Autodesk Inventor part; units mm, degrees
ref_plane "YZ Plane" through (0, 0, 0) normal (1, 0, 0) x (0, 1, 0)
ref_plane "XZ Plane" through (0, 0, 0) normal (0, 1, 0) x (-1, 0, 0)
ref_plane "XY Plane" through (0, 0, 0) normal (0, 0, 1) x (1, 0, 0)
sketch "Sketch1" plane through (0, 0, 0) normal (0, 0, 1) x (1, 0, 0)
  circle A0 centre (0, 0) radius 30
  circle A1 centre (0, 0) radius 22
  dimension "d0" = 60
  dimension "d1" = 44
extrude "Extrusion1" add sketch "Sketch1" against normal blind 1.17
sketch "Sketch2" plane through (0, 0, 0) normal (0, 0, 1) x (1, 0, 0)
  circle A0 centre (0, 0) radius 26 construction
  line L0 (-1.8, 24.6) -> (1.8, 24.6)
  line L1 (1.8, 24.6) -> (1.8, 27.4)
  line L2 (1.8, 27.4) -> (-1.8, 27.4)
  line L3 (-1.8, 27.4) -> (-1.8, 24.6)
  line L4 (-1.8, 24.6) -> (1.8, 27.4) construction
  line L5 (1.8, 24.6) -> (-1.8, 27.4) construction
  line L6 (12.789, 24.299) -> (9.5002, 25.7633)
  line L7 (11.6501, 21.7411) -> (12.789, 24.299)
  line L8 (8.3613, 23.2053) -> (11.6501, 21.7411)
  circle A1 centre (0, 0) radius 26 construction
  line L9 (9.5002, 25.7633) -> (8.3613, 23.2053)
  line L10 (21.5666, 16.9965) -> (19.1577, 19.6718)
  line L11 (19.4858, 15.123) -> (21.5666, 16.9965)
  line L12 (17.0769, 17.7983) -> (19.4858, 15.123)
  circle A2 centre (0, 0) radius 26 construction
  line L13 (19.1577, 19.6718) -> (17.0769, 17.7983)
  line L14 (26.6152, 6.7552) -> (25.5027, 10.179)
  line L15 (23.9522, 5.8899) -> (26.6152, 6.7552)
  line L16 (22.8398, 9.3137) -> (23.9522, 5.8899)
  circle A3 centre (0, 0) radius 26 construction
  line L17 (25.5027, 10.179) -> (22.8398, 9.3137)
  line L18 (27.0617, -4.6542) -> (27.4381, -1.0739)
  line L19 (24.2771, -4.3615) -> (27.0617, -4.6542)
  line L20 (24.6534, -0.7813) -> (24.2771, -4.3615)
  circle A4 centre (0, 0) radius 26 construction
  line L21 (27.4381, -1.0739) -> (24.6534, -0.7813)
  line L22 (22.8291, -15.2588) -> (24.6291, -12.1412)
  line L23 (20.4042, -13.8588) -> (22.8291, -15.2588)
  line L24 (22.2042, -10.7412) -> (20.4042, -13.8588)
  circle A5 centre (0, 0) radius 26 construction
  line L25 (24.6291, -12.1412) -> (22.2042, -10.7412)
  line L26 (14.6491, -23.2251) -> (17.5615, -21.1091)
  line L27 (13.0033, -20.9598) -> (14.6491, -23.2251)
  line L28 (15.9157, -18.8438) -> (13.0033, -20.9598)
  circle A6 centre (0, 0) radius 26 construction
  line L29 (17.5615, -21.1091) -> (15.9157, -18.8438)
  line L30 (3.9361, -27.1755) -> (7.4574, -26.427)
  line L31 (3.354, -24.4367) -> (3.9361, -27.1755)
  line L32 (6.8753, -23.6882) -> (3.354, -24.4367)
  circle A7 centre (0, 0) radius 26 construction
  line L33 (7.4574, -26.427) -> (6.8753, -23.6882)
  line L34 (-7.4574, -26.427) -> (-3.9361, -27.1755)
  line L35 (-6.8753, -23.6882) -> (-7.4574, -26.427)
  line L36 (-3.354, -24.4367) -> (-6.8753, -23.6882)
  circle A8 centre (0, 0) radius 26 construction
  line L37 (-3.9361, -27.1755) -> (-3.354, -24.4367)
  line L38 (-17.5615, -21.1091) -> (-14.6491, -23.2251)
  line L39 (-15.9157, -18.8438) -> (-17.5615, -21.1091)
  line L40 (-13.0033, -20.9598) -> (-15.9157, -18.8438)
  circle A9 centre (0, 0) radius 26 construction
  line L41 (-14.6491, -23.2251) -> (-13.0033, -20.9598)
  line L42 (-24.6291, -12.1412) -> (-22.8291, -15.2588)
  line L43 (-22.2042, -10.7412) -> (-24.6291, -12.1412)
  line L44 (-20.4042, -13.8588) -> (-22.2042, -10.7412)
  circle A10 centre (0, 0) radius 26 construction
  line L45 (-22.8291, -15.2588) -> (-20.4042, -13.8588)
  line L46 (-27.4381, -1.0739) -> (-27.0617, -4.6542)
  line L47 (-24.6534, -0.7813) -> (-27.4381, -1.0739)
  line L48 (-24.2771, -4.3615) -> (-24.6534, -0.7813)
  circle A11 centre (0, 0) radius 26 construction
  line L49 (-27.0617, -4.6542) -> (-24.2771, -4.3615)
  line L50 (-25.5027, 10.179) -> (-26.6152, 6.7552)
  line L51 (-22.8398, 9.3137) -> (-25.5027, 10.179)
  line L52 (-23.9522, 5.8899) -> (-22.8398, 9.3137)
  circle A12 centre (0, 0) radius 26 construction
  line L53 (-26.6152, 6.7552) -> (-23.9522, 5.8899)
  line L54 (-19.1577, 19.6718) -> (-21.5666, 16.9965)
  line L55 (-17.0769, 17.7983) -> (-19.1577, 19.6718)
  line L56 (-19.4858, 15.123) -> (-17.0769, 17.7983)
  circle A13 centre (0, 0) radius 26 construction
  line L57 (-21.5666, 16.9965) -> (-19.4858, 15.123)
  line L58 (-9.5002, 25.7633) -> (-12.789, 24.299)
  line L59 (-8.3613, 23.2053) -> (-9.5002, 25.7633)
  line L60 (-11.6501, 21.7411) -> (-8.3613, 23.2053)
  circle A14 centre (0, 0) radius 26 construction
  line L61 (-12.789, 24.299) -> (-11.6501, 21.7411)
  point P0 (0, 26)
  point P1 (10.5752, 23.7522)
  point P2 (19.3218, 17.3974)
  point P3 (24.7275, 8.0344)
  point P4 (25.8576, -2.7177)
  point P5 (22.5167, -13)
  point P6 (15.2824, -21.0344)
  point P7 (5.4057, -25.4318)
  point P8 (-5.4057, -25.4318)
  point P9 (-15.2824, -21.0344)
  point P10 (-22.5167, -13)
  point P11 (-25.8576, -2.7177)
  point P12 (-24.7275, 8.0344)
  point P13 (-19.3218, 17.3974)
  point P14 (-10.5752, 23.7522)
  dimension "d4" = 52
  dimension "d5" = 3.6
  dimension "d6" = 2.8
  dimension "d9" = 360
extrude "Extrusion2" add sketch "Sketch2" along normal blind 1.6
properties part number "AndyMarkLightRing2018"
Can you work these out from the model? Positions are in its coordinate system, mm. A direction names the side the tool comes from. Give positions to 0.01 mm unless a question says otherwise; leave off trailing zeros. Loops run counter-clockwise (first coordinate to the right, second up) from the corner with the lowest first, then second, coordinate; pieces in that order, holes last. Notation, with made-up numbers: M -40,49.25 L -12,49.25 A7 cw -12,58.25 Z; hole C 38,14.25 d7. An arc over 180 degrees is marked long. One line per item, written item: value. Start each with the question number.
1) If we section it at B-B, the plane x = 0: Write out the boundary of the cut face in (y, z).
2) If we section it at C-C, the plane z = 0.9: Give the number of separate pieces and of enclosed holes in the cut face, and give its area (3 significant figures).
3) Thinking about a two-plate mould opening in X: for faces 6 (the face through (-26.026, -0.926, 0.789)), 7 (the face through (5, -25, 1.6)), 8 (the face through (-3.65, -25.83, 0.79)), which applies, +X half, -X half, draft (parallel to the pull), parting line (faces both ways), or undercut?
4) On a 3-axis mill with a long thin cutter (end or side, diameter ignored), from which of +Z, -Z, +X, -X, +Y, -Y can I reach the whole of each face in a straight line? I mean faces 1 (the face through (-23.404, 7.578, 0.789)), 2 (the face through (-23.74, -13.68, 0.79)), 3 (the face through (-25.302, 6.329, 0.789)), 4 (the face through (-18.1, 18.72, 0.79)), 5 (the face through (-13.84, -22.11, 0.79)). Say none if no direction works.
5) I'm going to push flat-ended pins straight in: pin 1 (1.3 mm diameter, centred on x = -0.5, z = 0.5, fed in from +Y); pin 2 (2 mm diameter, centred on x = 10, y = -19.5, fed in from +Z); pin 3 (0.8 mm diameter, centred on y = 26, z = 1, fed in from -X); pin 4 (5 mm diameter, centred on x = -17.5, y = -6.5, fed in from +Z). Where does each tip first touch, or does it pass through?
6) If we section it at A-A, the plane y = 0: Write out the boundary of the cut face in (x, z), and give its area (3 significant figures).
7) If I drill on line 1 (Y direction, x = 0, z = -0.4); line 2 (Z direction, x = 25.5, y = -15); line 3 (Y direction, x = 6, z = -0.95), over which ranges is the centre line in solid material (lowest first)? Write a range as [from, to].
Completed:
1. outline: M -30,-1.17 L -22,-1.17 L -22,0 L -30,0 Z; M 22,-1.17 L 30,-1.17 L 30,0 L 27.4,0 L 27.4,1.6 L 24.6,1.6 L 24.6,0 L 22,0 Z
2. separate pieces: 15
2. enclosed holes: 0
2. area: 151 mm^2
3. face 6: -X half
3. face 7: draft
3. face 8: undercut
4. face 1: +Z
4. face 2: +Z, -X, -Y
4. face 3: +Z, -X
4. face 4: +Z, +Y
4. face 5: +Z, -Y
5. pin 1: stops at y = 30
5. pin 2: stops at z = 0
5. pin 3: stops at x = -9.87
5. pin 4: passes through
6. outline: M -30,-1.17 L -22,-1.17 L -22,0 L -30,0 Z; M 22,-1.17 L 30,-1.17 L 30,0 L 22,0 Z
6. area: 18.7 mm^2
7. line 1: y = [-30, -22], [22, 30]
7. line 2: z = [-1.17, 0]
7. line 3: y = [-29.39, -21.17], [21.17, 29.39]
